Read the model definition and answer for the solid it produces. Units are mm, in the model's axes. Coordinates: 2 decimals unless noted, no trailing zeros. Write each loop counter-clockwise with the first axis right and the second up, starting at its lowest first coordinate (ties: lowest second). Pieces come first, ordered by that corner, then holes. Notation, with made-up numbers: (49, -9.5) -> (107, -9.5) arc R9 cw to (107, -2.5) -> close; hole circle Ø7 at (6, 60.5). An arc over 180 degrees is marked (long way). Return JSON: item names as keys, results as strings.
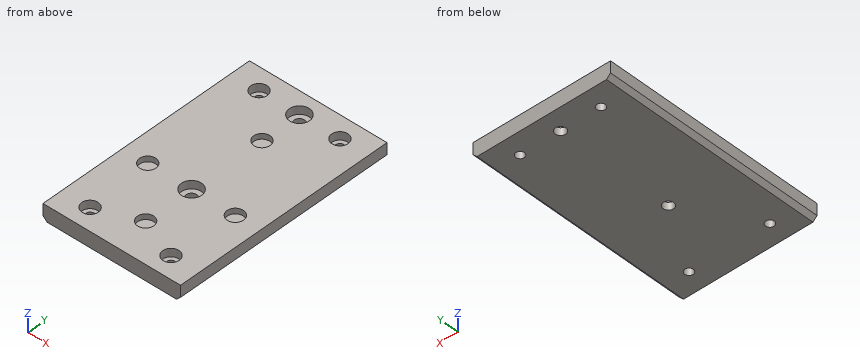
from build123d import *

# Parameters (mm, degrees)
SKETCH1_W           = 68
SKETCH1_H           = 110
SKETCH1_R           = 2.1
SKETCH1_R_2         = 4.05
SKETCH1_R_3         = 2.6
BOSS_EXTRUDE1_DEPTH = 7.7
SKETCH2_R           = 6.304633146
SKETCH2_R_2         = 7.334333348
SKETCH2_R_3         = 8.114040952
SKETCH2_R_4         = 11.073656437
BOSS_EXTRUDE2_DEPTH = 5
SKETCH3_R           = 4.05
SKETCH3_R_2         = 5
CUT_EXTRUDE1_DEPTH  = 4
CUT_EXTRUDE2_DEPTH  = 111


with BuildPart() as part:
    # Sketch1 → Boss-Extrude1 (new body)
    with BuildSketch(Plane.XY):
        Rectangle(SKETCH1_W, SKETCH1_H)
        with Locations((20, 45)):
            Circle(SKETCH1_R, mode=Mode.SUBTRACT)
        with Locations((-20, 45)):
            Circle(SKETCH1_R, mode=Mode.SUBTRACT)
        with Locations((20, -45)):
            Circle(SKETCH1_R, mode=Mode.SUBTRACT)
        with Locations((-20, -45)):
            Circle(SKETCH1_R, mode=Mode.SUBTRACT)
        with Locations((21.650635095, -12.5)):
            Circle(SKETCH1_R_2, mode=Mode.SUBTRACT)
        with Locations((0, 25)):
            Circle(SKETCH1_R_2, mode=Mode.SUBTRACT)
        with Locations((-21.650635095, -12.5)):
            Circle(SKETCH1_R_2, mode=Mode.SUBTRACT)
        with Locations((0, -36.95)):
            Circle(SKETCH1_R_2, mode=Mode.SUBTRACT)
        with Locations((0, 45)):
            Circle(SKETCH1_R_3, mode=Mode.SUBTRACT)
        with Locations((0, -12.5)):
            Circle(SKETCH1_R_3, mode=Mode.SUBTRACT)
    extrude(amount=BOSS_EXTRUDE1_DEPTH)

    # Sketch2 → Boss-Extrude2 (add)
    with BuildSketch(Plane(origin=(0, 0, 0), x_dir=(-1, 0, 0), z_dir=(0, 0, -1))):
        with Locations((-21.650635095, -12.5)):
            Circle(SKETCH2_R)
        with Locations((0, 25)):
            Circle(SKETCH2_R_2)
        with Locations((21.650635095, -12.5)):
            Circle(SKETCH2_R_3)
        with Locations((0, -36.95)):
            Circle(SKETCH2_R_4)
    extrude(amount=-BOSS_EXTRUDE2_DEPTH)

    # Sketch3 → Cut-Extrude1 (cut)
    with BuildSketch(Plane(origin=(0, 0, 7.7), x_dir=(-1, 0, 0), z_dir=(0, 0, -1))):
        with Locations((-20, 45)):
            Circle(SKETCH3_R)
        with Locations((20, 45)):
            Circle(SKETCH3_R)
        with Locations((-20, -45)):
            Circle(SKETCH3_R)
        with Locations((20, -45)):
            Circle(SKETCH3_R)
        with Locations((0, 45)):
            Circle(SKETCH3_R_2)
        with Locations((0, -12.5)):
            Circle(SKETCH3_R_2)
    extrude(amount=CUT_EXTRUDE1_DEPTH, mode=Mode.SUBTRACT)

    # Sketch4 → Cut-Extrude2 (cut, through all)
    with BuildSketch(Plane.XZ.offset(55)):
        Polygon((34, 2), (34, 0), (32, 0), align=None)
        Polygon((-34, 15.4), (-39, 15.4), (-39, 0), (-34, 0), (-32, 0), (-34, 2), align=None)
    extrude(amount=-CUT_EXTRUDE2_DEPTH, mode=Mode.SUBTRACT)


solid = part.part
1. The part is cut by section B-B (y = -45). Determine the outline of the cut face in (x, z), then the cut area to 3 significant figures.
Taken from the geometry:
{"outline": "(-34, 2) -> (-32, 0) -> (-22.1, 0) -> (-22.1, 3.7) -> (-24.05, 3.7) -> (-24.05, 7.7) -> (-34, 7.7) -> close; (-17.9, 0) -> (17.9, 0) -> (17.9, 3.7) -> (15.95, 3.7) -> (15.95, 7.7) -> (-15.95, 7.7) -> (-15.95, 3.7) -> (-17.9, 3.7) -> close; (22.1, 0) -> (32, 0) -> (34, 2) -> (34, 7.7) -> (24.05, 7.7) -> (24.05, 3.7) -> (22.1, 3.7) -> close", "area": "424 mm2"}
2. Consider L1, parallel to Y at x = 0, z = 6.7; L2, parallel to Y at x = 20, z = 1.4; L3, parallel to Y at x = 3, z = 5.5. Determine where each line is inside the solid, lowest interval first.
Taken from the geometry:
{"L1": "y = -55 to -41, -32.9 to -17.5, -7.5 to 20.95, 29.05 to 40, 50 to 55", "L2": "y = -55 to -47.1, -42.9 to 42.9, 47.1 to 55", "L3": "y = -55 to -39.67, -34.23 to -16.5, -8.5 to 22.28, 27.72 to 41, 49 to 55"}
3. The part is cut by section A-A (y = -12.5). Determine the outline of the cut face in (x, z), then the cut area to 3 significant figures.
Taken from the geometry:
{"outline": "(-34, 2) -> (-32, 0) -> (-2.6, 0) -> (-2.6, 3.7) -> (-5, 3.7) -> (-5, 7.7) -> (-17.6, 7.7) -> (-17.6, 5) -> (-25.7, 5) -> (-25.7, 7.7) -> (-34, 7.7) -> close; (2.6, 0) -> (32, 0) -> (34, 2) -> (34, 7.7) -> (25.7, 7.7) -> (25.7, 5) -> (17.6, 5) -> (17.6, 7.7) -> (5, 7.7) -> (5, 3.7) -> (2.6, 3.7) -> close", "area": "417 mm2"}
4. The part is cut by section C-C (x = 20). Determine the outline of the cut face in (y, z), then the cut area to 3 significant figures.
Taken from the geometry:
{"outline": "(-55, 0) -> (-47.1, 0) -> (-47.1, 3.7) -> (-49.05, 3.7) -> (-49.05, 7.7) -> (-55, 7.7) -> close; (-42.9, 0) -> (42.9, 0) -> (42.9, 3.7) -> (40.95, 3.7) -> (40.95, 7.7) -> (-8.8, 7.7) -> (-8.8, 5) -> (-16.2, 5) -> (-16.2, 7.7) -> (-40.95, 7.7) -> (-40.95, 3.7) -> (-42.9, 3.7) -> close; (47.1, 0) -> (55, 0) -> (55, 7.7) -> (49.05, 7.7) -> (49.05, 3.7) -> (47.1, 3.7) -> close", "area": "731 mm2"}
5. Flat-ended cylindrical pins translate along their axes: pin 1 Ø4 at (x, y) = (-19.5, -46.5) entering from +Z; pin 2 Ø5 at (x, y) = (21.65, -12.5) entering from -Z. Find the tip coordinate at first contact, or state that the pin passes through.
Taken from the geometry:
{"pin 1": "stops at z = 3.7", "pin 2": "stops at z = 0"}
